```python
from build123d import *

# Parameters (mm, degrees)
SKETCH1_R                       = 15.875
SKETCH1_R_2                     = 12.7
INITIAL_PLATE_DEPTH             = 3.175
SKETCH2_R                       = 2.54
INITIAL_HOLE_FRONT_DEPTH        = 4.175
FRONT_SUPPORT_MOUNTS_COUNT      = 2
FRONT_SUPPORT_MOUNTS_PITCH      = 28.575
SKETCH3_R                       = 2.54
MAX_PLANETARY_HOLES_DEPTH       = 4.175
MAX_PLANETARY_PATTERN_COUNT     = 3
MAX_PLANETARY_PATTERN_ANGLE     = 180
SKETCH4_R                       = 2.54
INITIAL_STATIC_HOOD_MOUNT_DEPTH = 4.175
HOOD_MOUNTING_PATTERN_COUNT     = 4
HOOD_MOUNTING_PATTERN_ANGLE     = 30
SKETCH5_R                       = 2.54
INITIAL_MOUNTING_HOLE_DEPTH     = 4.175
MOUNTING_PATTERN_COUNT          = 6
MOUNTING_PATTERN_PITCH          = 25.4
SKETCH6_R                       = 2.54
BEARING_RETAINER_MOUNT_DEPTH    = 4.175


with BuildPart() as part:
    # Sketch1 → Initial Plate (new body)
    with BuildSketch(Plane(origin=(0, 0, 0), x_dir=(1, 0, 0), z_dir=(0, 1, 0))):
        with BuildLine():
            Line((-186.6511184, 50.8), (56.888798458, 50.8))
            ThreePointArc((56.888798458, 50.8), (62.753005846, 49.365037581), (67.29202942, 45.384420742))
            Line((67.29202942, 45.384420742), (114.89294907, -22.596737775))
            ThreePointArc((114.89294907, -22.596737775), (117.478368927, -62.042622164), (83.683256183, -82.55))
            Line((83.683256183, -82.55), (-190.5, -82.55))
            ThreePointArc((-190.5, -82.55), (-199.480256121, -78.830256121), (-203.2, -69.85))
            Line((-203.2, -69.85), (-203.2, 0))
            ThreePointArc((-203.2, 0), (-202.171026291, 20.423421079), (-199.094526293, 40.64))
            ThreePointArc((-199.094526293, 40.64), (-194.683303657, 47.937377699), (-186.6511184, 50.8))
        make_face()
        Circle(SKETCH1_R, mode=Mode.SUBTRACT)
        with Locations((76.989658396, -44.45)):
            Circle(SKETCH1_R_2, mode=Mode.SUBTRACT)
    extrude(amount=INITIAL_PLATE_DEPTH)

    # Sketch2 → Initial Hole Front (cut, through all)
    with BuildSketch(Plane(origin=(0, 3.175, 0), x_dir=(1, 0, 0), z_dir=(0, 1, 0))):
        with Locations((55.280583464, 40.396769038)):
            Circle(SKETCH2_R)
    initial_hole_front = extrude(amount=-INITIAL_HOLE_FRONT_DEPTH, mode=Mode.SUBTRACT)

    # Front Support Mounts: Initial Hole Front ×2
    with Locations(*[Vector(0.573576436, 0, 0.819152044) * (i * FRONT_SUPPORT_MOUNTS_PITCH) for i in range(1, FRONT_SUPPORT_MOUNTS_COUNT)]):
        add(initial_hole_front, mode=Mode.SUBTRACT)

    # Sketch3 → Max Planetary Holes (cut, through all)
    with BuildSketch(Plane(origin=(0, 3.175, 0), x_dir=(1, 0, 0), z_dir=(0, 1, 0))):
        with Locations((59.029146154, -26.489487758)):
            Circle(SKETCH3_R)
        with Locations((102.389658396, -44.45)):
            Circle(SKETCH3_R)
        with Locations((94.950170639, -62.410512242)):
            Circle(SKETCH3_R)
        with Locations((51.589658396, -44.45)):
            Circle(SKETCH3_R)
    max_planetary_holes = extrude(amount=-MAX_PLANETARY_HOLES_DEPTH, mode=Mode.SUBTRACT)

    # Max Planetary Pattern: Max Planetary Holes ×3 about axis
    max_planetary_pattern_axis = Axis((76.989658396, 0, 44.45), (0, 1, 0))
    for i in range(1, MAX_PLANETARY_PATTERN_COUNT):
        add(max_planetary_holes.rotate(max_planetary_pattern_axis, i * MAX_PLANETARY_PATTERN_ANGLE / (MAX_PLANETARY_PATTERN_COUNT - 1)), mode=Mode.SUBTRACT)

    # Sketch4 → Initial Static Hood Mount (cut, through all)
    with BuildSketch(Plane(origin=(0, 3.175, 0), x_dir=(1, 0, 0), z_dir=(0, 1, 0))):
        with Locations((-186.339919668, 39.593993711)):
            Circle(SKETCH4_R)
    initial_static_hood_mount = extrude(amount=-INITIAL_STATIC_HOOD_MOUNT_DEPTH, mode=Mode.SUBTRACT)

    # Hood Mounting Pattern: Initial Static Hood Mount ×4 about axis
    hood_mounting_pattern_axis = Axis((0, 0, 0), (0, 1, 0))
    for i in range(1, HOOD_MOUNTING_PATTERN_COUNT):
        add(initial_static_hood_mount.rotate(hood_mounting_pattern_axis, i * HOOD_MOUNTING_PATTERN_ANGLE / (HOOD_MOUNTING_PATTERN_COUNT - 1)), mode=Mode.SUBTRACT)

    # Sketch5 → Initial Mounting Hole (cut, through all)
    with BuildSketch(Plane(origin=(0, 3.175, 0), x_dir=(1, 0, 0), z_dir=(0, 1, 0))):
        with Locations((-139.7, -69.85)):
            Circle(SKETCH5_R)
    initial_mounting_hole = extrude(amount=-INITIAL_MOUNTING_HOLE_DEPTH, mode=Mode.SUBTRACT)

    # Mounting Pattern: Initial Mounting Hole ×6
    with Locations(*[(i * MOUNTING_PATTERN_PITCH, 0, 0) for i in range(1, MOUNTING_PATTERN_COUNT)]):
        add(initial_mounting_hole, mode=Mode.SUBTRACT)

    # Sketch6 → Bearing Retainer Mount (cut, through all)
    with BuildSketch(Plane(origin=(0, 3.175, 0), x_dir=(1, 0, 0), z_dir=(0, 1, 0))):
        with Locations((-20.205576272, 20.205576272)):
            Circle(SKETCH6_R)
        with Locations((20.205576272, -20.205576272)):
            Circle(SKETCH6_R)
    extrude(amount=-BEARING_RETAINER_MOUNT_DEPTH, mode=Mode.SUBTRACT)


solid = part.part
```
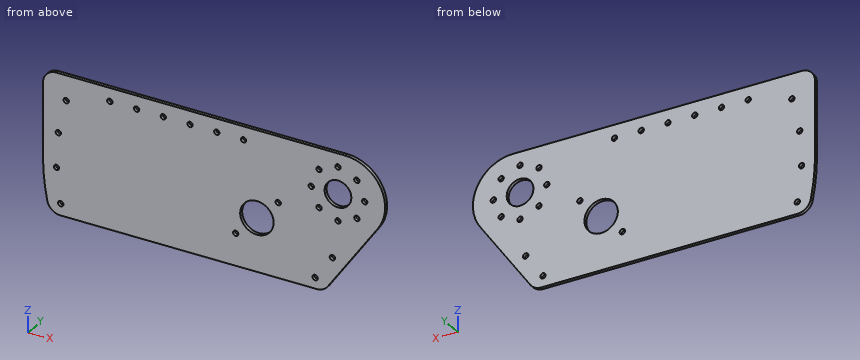
Can you work these out from the model? Positions are in its coordinate system, mm. Coordinates: 2 decimals unless noted, no trailing zeros. Loops run counter-clockwise (first coordinate to the right, second up) from the corner with the lowest first, then second, coordinate; pieces in that order, holes last. Notation, with made-up numbers: (46.5, -37) - (103.5, -37) arc R18 cw to (103.5, -31) - close; hole circle Ø11 at (43, 4.5). An arc over 180 degrees is marked (long way). Use a Markdown table: item, result.
Item 1: I want a section at C-C on z = 35. Please give me the cut outline in (x, y) (3 decimals), and give its area (3 significant figures).
Numbers:
| item | result |
|---|---|
| outline | (-203.2, 0) - (68.505, 0) - (68.505, 3.175) - (-203.2, 3.175) - close; (85.474, 0) - (120.593, 0) - (120.593, 3.175) - (85.474, 3.175) - close |
| area | 974 mm2 |
Item 2: I want a section at B-B on y = 0.5. Give the number of separate pieces and of enclosed holes in the cut face, and give its area (3 significant figures).
Numbers:
| item | result |
|---|---|
| separate pieces | 1 |
| enclosed holes | 24 |
| area | 38,700 mm2 |
Item 3: If I drill on probe 1 along Z at (x, y) = (76, 2.45); probe 2 along X at (y, z) = (0.15, 63.5); probe 3 along X at (y, z) = (2.3, 19), over which ranges is the centre line in solid material (lowest first)? Write a range as from..to.
Numbers:
| item | result |
|---|---|
| probe 1 | z = -32.95..16.71, 21.39..31.79, 57.11..67.51, 72.19..82.55 |
| probe 2 | x = -203.2..56.73, 61.32..92.66, 97.24..116.68 |
| probe 3 | x = -203.2..17.97, 22.44..74.45, 79.53..112.37 |
Item 4: I want a section at D-D on z = -26.5. Please give me the cut outline in (x, y) (3 decimals), and give its area (3 significant figures).
Numbers:
| item | result |
|---|---|
| outline | (-201.465, 0) - (80.515, 0) - (80.515, 3.175) - (-201.465, 3.175) - close |
| area | 895 mm2 |
Item 5: I want a section at A-A on z = 10.5. Please give me the cut outline in (x, y) (3 decimals).
Numbers:
| item | result |
|---|---|
| outline | (-203.2, 0) - (-11.907, 0) - (-11.907, 3.175) - (-203.2, 3.175) - close; (11.907, 0) - (106.423, 0) - (106.423, 3.175) - (11.907, 3.175) - close |
